Geometry check sheet. Reference: the model listing, model coordinates, mm. A direction names the side the tool comes from. Give positions to 0.01 mm unless a question says otherwise; leave off trailing zeros. Order: outer loops, then holes, each group sorted by start corner. A loop starts at its lowest first (then second) coordinate and runs counter-clockwise, first axis right, second up. Notation, with made-up numbers: M -26,-33.5 L -11,-33.5 A30 ccw -11,-11.5 Z; hole C -27.75,-1.5 d11. An arc over 180 degrees is marked long. Answer as CSV lines item,"result". Start each with the question number.
Q1. Mould release check, pull along Y, two halves, no side actions. Record for faces 3 (the cylindrical face through (97.15, -96.99, -0.14)), 4 (the flat face through (1, 1, -10)), 5 (the flat face through (-72.8, 72.8, 4)): +Y half, -Y half, draft (parallel to the pull), parting line (faces both ways), or undercut.
Q2. Section check D-D, the plane y = -27. Record the boundary of the cut face in (x, z), then the cut area to 3 significant figures.
Q3. Thickness scan on line 1 (Y direction, x = -75, z = 8.15); line 2 (Y direction, x = 75, z = -6.5); line 3 (Y direction, x = 0, z = 5.75). Record the ranges inside material, lowest first.
Q4. Section check C-C, the plane x = 0. Record the boundary of the cut face in (y, z).
Q5. Set-up check for faces 1 (the cylindrical face through (72.253, 75.121, -2.902)), 2 (the cylindrical face through (79.619, -76.915, 7.042)): record each of +Z, -Z, +X, -X, +Y, -Y from which the full face is reachable in a straight line by a thin tool's end or side.
Q6. Go/stop test with flat-tipped pins: pin 1 (5.5 mm diameter, centred on x = 27.5, y = 47.63, fed in from +Z); pin 2 (3 mm diameter, centred on x = -77, y = -73, fed in from +Z); pin 3 (2.5 mm diameter, centred on x = 27.5, y = -47.63, fed in from +Z). Record where each tip stops, or that it passes through.
Q7. Section check A-A, the plane x = 75. Record the boundary of the cut face in (y, z).
```python
from build123d import *

# Parameters (mm, degrees)
SKETCH_1_W          = 200
SKETCH_1_H          = 200
SKETCH_1_R          = 63
EXTRUDE_1_DEPTH     = 10
SKETCH_2_W          = 200
SKETCH_2_H          = 200
EXTRUDE_2_DEPTH     = 10
SKETCH_3_R          = 2.1
CUT_EXTRUDE_1_DEPTH = 10
SKETCH_4_R          = 2.75
CUT_EXTRUDE_2_DEPTH = 143.828568571
SKETCH_5_R          = 5
CUT_EXTRUDE_3_DEPTH = 6
FILLET_1_R          = 10


with BuildPart() as part:
    # ｽｹｯﾁ1 → ﾎﾞｽ - 押し出し1 (new body)
    with BuildSketch(Plane.XY):
        Rectangle(SKETCH_1_W, SKETCH_1_H)
        Circle(SKETCH_1_R, mode=Mode.SUBTRACT)
    extrude(amount=EXTRUDE_1_DEPTH)

    # ｽｹｯﾁ2 → ﾎﾞｽ - 押し出し2 (add)
    with BuildSketch(Plane(origin=(0, 0, 0), x_dir=(-1, 0, 0), z_dir=(0, 0, -1))):
        Rectangle(SKETCH_2_W, SKETCH_2_H)
    extrude(amount=EXTRUDE_2_DEPTH)

    # ｽｹｯﾁ3 → ｶｯﾄ - 押し出し1 (cut)
    with BuildSketch(Plane.XY):
        with Locations((27.5, -47.631397208)):
            Circle(SKETCH_3_R)
        with Locations((-27.5, -47.631397208)):
            Circle(SKETCH_3_R)
        with Locations((-55, 0)):
            Circle(SKETCH_3_R)
        with Locations((-27.5, 47.631397208)):
            Circle(SKETCH_3_R)
        with Locations((27.5, 47.631397208)):
            Circle(SKETCH_3_R)
        with Locations((55, 0)):
            Circle(SKETCH_3_R)
    extrude(amount=-CUT_EXTRUDE_1_DEPTH, mode=Mode.SUBTRACT)

    # ｽｹｯﾁ4 → ｶｯﾄ - 押し出し2 (cut, through all)
    with BuildSketch(Plane.XY.offset(10)):
        with Locations((75, 75)):
            Circle(SKETCH_4_R)
        with Locations((75, -75)):
            Circle(SKETCH_4_R)
        with Locations((-75, -75)):
            Circle(SKETCH_4_R)
        with Locations((-75, 75)):
            Circle(SKETCH_4_R)
    extrude(amount=-CUT_EXTRUDE_2_DEPTH, mode=Mode.SUBTRACT)

    # ｽｹｯﾁ5 → ｶｯﾄ - 押し出し3 (cut)
    with BuildSketch(Plane.XY.offset(10)):
        with Locations((75, -75)):
            Circle(SKETCH_5_R)
        with Locations((-75, -75)):
            Circle(SKETCH_5_R)
        with Locations((-75, 75)):
            Circle(SKETCH_5_R)
        with Locations((75, 75)):
            Circle(SKETCH_5_R)
    extrude(amount=-CUT_EXTRUDE_3_DEPTH, mode=Mode.SUBTRACT)

    # ﾌｨﾚｯﾄ1
    fillet_1_edges = [part.edges().sort_by_distance(p)[0] for p in [
        (100, -100, 0),
        (-100, -100, 0),
        (-100, 100, 0),
        (100, 100, 0),
    ]]
    fillet(fillet_1_edges, radius=FILLET_1_R)


solid = part.part
```
Answer block:
1,face 3,"-Y half"
1,face 4,"draft"
1,face 5,"undercut"
2,outline,"M -100,-10 L 100,-10 L 100,10 L 56.92,10 L 56.92,0 L -56.92,0 L -56.92,10 L -100,10 Z"
2,area,"2,860 mm2"
3,line 1,"y = -100 to -80, -70 to 70, 80 to 100"
3,line 2,"y = -100 to -77.75, -72.25 to 72.25, 77.75 to 100"
3,line 3,"y = -100 to -63, 63 to 100"
4,outline,"M -100,-10 L 100,-10 L 100,10 L 63,10 L 63,0 L -63,0 L -63,10 L -100,10 Z"
5,face 1,"+Z, -Z"
5,face 2,"+Z"
6,pin 1,"stops at z = 0"
6,pin 2,"stops at z = 4"
6,pin 3,"passes through"
7,outline,"M -100,-10 L -77.75,-10 L -77.75,4 L -80,4 L -80,10 L -100,10 Z; M -72.25,-10 L 72.25,-10 L 72.25,4 L 70,4 L 70,10 L -70,10 L -70,4 L -72.25,4 Z; M 77.75,-10 L 100,-10 L 100,10 L 80,10 L 80,4 L 77.75,4 Z"
